Can you work these out from the model? Positions are in its coordinate system, mm. Face numbers are marked on the shaded views. Round coordinates to 2 decimals unless told otherwise and drop trailing zeros. Loops run counter-clockwise (first coordinate to the right, second up) from the corner with the lowest first, then second, coordinate; pieces in that order, holes last. Notation, with made-up numbers: M -27,8 L -13,8 A18 cw -13,35 Z; hole C -16.75,64.5 d5. An arc over 180 degrees is marked long. Use a Markdown table: item, result. Add a question column.
```python
from build123d import *

# Parameters (mm, degrees)
BOSS_EXTRUDE1_DEPTH = 3
BOSS_EXTRUDE2_DEPTH = 1
SKETCH2_R           = 1
CUT_EXTRUDE1_DEPTH  = 4


with BuildPart() as part:
    # Sketch1 → Boss-Extrude1 (new body)
    with BuildSketch(Plane.XY):
        with BuildLine():
            Line((0, 83), (0, 6))
            ThreePointArc((0, 6), (1.757359313, 1.757359313), (6, 0))
            ThreePointArc((6, 0), (10.242640687, 1.757359313), (12, 6))
            Line((12, 6), (12, 83))
            Line((12, 83), (0, 83))
        make_face()
        with BuildLine():
            Line((1.882949163, 6.83059762), (3.675, 24.775))
            ThreePointArc((3.675, 24.775), (6, 27.1), (8.325, 24.775))
            Line((8.325, 24.775), (10.117050837, 6.83059762))
            ThreePointArc((10.117050837, 6.83059762), (6, 1.8), (1.882949163, 6.83059762))
        make_face(mode=Mode.SUBTRACT)
    extrude(amount=BOSS_EXTRUDE1_DEPTH)

    # Sketch1_3 → Boss-Extrude2 (add)
    with BuildSketch(Plane.XY):
        with BuildLine():
            Line((0, 83), (0, 6))
            ThreePointArc((0, 6), (1.757359313, 1.757359313), (6, 0))
            ThreePointArc((6, 0), (10.242640687, 1.757359313), (12, 6))
            Line((12, 6), (12, 83))
            Line((12, 83), (0, 83))
        make_face()
        with BuildLine():
            Line((1.882949163, 6.83059762), (3.675, 24.775))
            ThreePointArc((3.675, 24.775), (6, 27.1), (8.325, 24.775))
            Line((8.325, 24.775), (10.117050837, 6.83059762))
            ThreePointArc((10.117050837, 6.83059762), (6, 1.8), (1.882949163, 6.83059762))
        make_face(mode=Mode.SUBTRACT)
        with BuildLine():
            ThreePointArc((8.325, 24.775), (6, 27.1), (3.675, 24.775))
            Line((3.675, 24.775), (1.882949163, 6.83059762))
            ThreePointArc((1.882949163, 6.83059762), (6, 1.8), (10.117050837, 6.83059762))
            Line((10.117050837, 6.83059762), (8.325, 24.775))
        make_face()
    extrude(amount=BOSS_EXTRUDE2_DEPTH)

    # Sketch2 → Cut-Extrude1 (cut, through all)
    with BuildSketch(Plane.XY.offset(3)):
        with BuildLine():
            Line((0, 83), (0, 77))
            ThreePointArc((0, 77), (1.757359313, 81.242640687), (6, 83))
            Line((6, 83), (0, 83))
        make_face()
        with BuildLine():
            Line((12, 83), (6, 83))
            ThreePointArc((6, 83), (10.242640687, 81.242640687), (12, 77))
            Line((12, 77), (12, 83))
        make_face()
        with Locations((6, 81)):
            Circle(SKETCH2_R)
    extrude(amount=-CUT_EXTRUDE1_DEPTH, mode=Mode.SUBTRACT)


solid = part.part
```
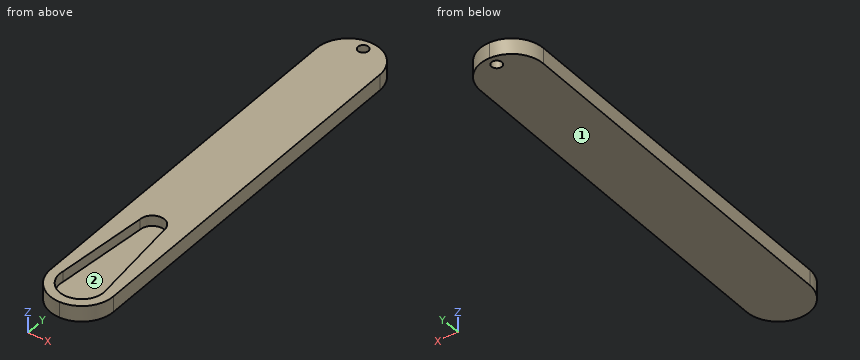
(1) I'm going to push a flat-ended pin straight in: pin 1 (4 mm diameter, centred on x = 4.5, y = 33.5, fed in from -Z). Where does the tip first touch, or does it pass through?
(2) Suppose I cut it at B-B on y = 81. List the corners of the cut face in (x, z) for me.
(3) Suppose I cut it at A-A on z = 2.05. List the corners of the cut face in (x, y) for me (3 decimals).
(4) Suppose I cut it at C-C on x = 2.75. List the corners of the cut face in (y, z) for me.
(5) Suppose I cut it at D-D on x = 9. List the corners of the cut face in (y, z) for me.
(6) Thinking about a two-plate mould opening in X: for the marked faces 1 and 2, which applies, released by +X, released by -X, zero draft, split by the parting line, or undercut?
(7) If I drill on probe 1 along X at (y, z) = (6, 2.45); probe 2 along X at (y, z) = (7, 1.8); probe 3 along Z at (x, y) = (6.75, 10), over which ranges is the centre line in solid material (lowest first)? Write a range as [from, to].
Results below:
| question | item | result |
|---|---|---|
| 1 | pin 1 | stops at z = 0 |
| 2 | outline | M 1.53,0 L 5,0 L 5,3 L 1.53,3 Z; M 7,0 L 10.47,0 L 10.47,3 L 7,3 Z |
| 3 | outline | M 0,6 A6 ccw 12,6 L 12,77 A6 ccw 0,77 Z; hole M 1.883,6.831 A4.2 ccw long 10.117,6.831 L 8.325,24.775 A2.325 ccw 3.675,24.775 Z; hole C 6,81 d2 |
| 4 | outline | M 0.96,0 L 82.04,0 L 82.04,3 L 15.51,3 L 15.51,1 L 3.34,1 L 3.34,3 L 0.96,3 Z |
| 5 | outline | M 0.8,0 L 82.2,0 L 82.2,3 L 18.02,3 L 18.02,1 L 3.06,1 L 3.06,3 L 0.8,3 Z |
| 6 | face 1 | zero draft |
| 6 | face 2 | undercut |
| 7 | probe 1 | x = [0, 1.8], [10.2, 12] |
| 7 | probe 2 | x = [0, 1.9], [10.1, 12] |
| 7 | probe 3 | z = [0, 1] |
